Read the model definition and answer for the solid it produces. Units are mm, in the model's axes. Round coordinates to 2 decimals unless told otherwise and drop trailing zeros. Loops run counter-clockwise (first coordinate to the right, second up) from the corner with the lowest first, then second, coordinate; pieces in that order, holes last. Notation, with made-up numbers: M 84,-29 L 109,-29 A32 cw 109,9 Z; hole C 16.5,45 d3. An arc over 180 degrees is marked long. Write each question's results on one line, items separated by ' | '.
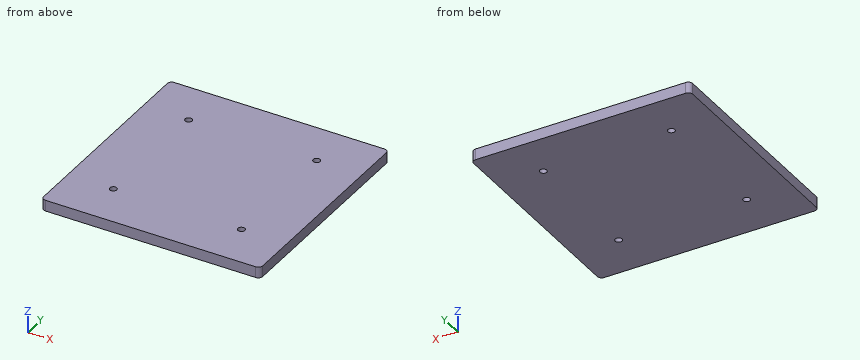
Autodesk Inventor part; units mm, degrees
ref_plane "YZ Plane" through (0, 0, 0) normal (1, 0, 0) x (0, 1, 0)
ref_plane "XZ Plane" through (0, 0, 0) normal (0, 1, 0) x (-1, 0, 0)
ref_plane "XY Plane" through (0, 0, 0) normal (0, 0, 1) x (1, 0, 0)
ref_plane "Plano de trabajo1" through (0, 0, 150) normal (0, 0, 1) x (1, 0, 0)
sketch "Boceto1" plane through (0, 0, 150) normal (0, 0, 1) x (1, 0, 0)
  line L0 (-96, 100) -> (96, 100)
  line L1 (100, 96) -> (100, -96)
  line L2 (96, -100) -> (-96, -100)
  line L3 (-100, -96) -> (-100, 96)
  line L4 (-100, 100) -> (100, -100) construction
  line L5 (100, 100) -> (-100, -100) construction
  arc A0 (100, 96) -> (96, 100) centre (96, 96) ccw
  arc A1 (-96, 100) -> (-100, 96) centre (-96, 96) ccw
  arc A2 (-100, -96) -> (-96, -100) centre (-96, -96) ccw
  arc A3 (96, -100) -> (100, -96) centre (96, -96) ccw
  circle A4 centre (58.5, 58.5) radius 3.175
  circle A5 centre (-58.5, 58.5) radius 3.175
  circle A6 centre (-58.5, -58.5) radius 3.175
  circle A7 centre (58.5, -58.5) radius 3.175
  point P0 (0, 0)
  dimension "d0" = 200
  dimension "d1" = 200
  dimension "d2" = 4
extrude "Extrusión1" add sketch "Boceto1" along normal blind 10
properties part number "TablaSoporte2" material "Madera (abedul)"
1. Find section A-A, the plane y = -58.5. Give the vertices of the cut face in (x, z) (3 decimals), then the cut area to 3 significant figures.
Completed:
outline: M -100,150 L -61.675,150 L -61.675,160 L -100,160 Z; M -55.325,150 L 55.325,150 L 55.325,160 L -55.325,160 Z; M 61.675,150 L 100,150 L 100,160 L 61.675,160 Z | area: 1,870 mm2
2. Find the intervals of material crossed by L1, parallel to Y at x = 58.5, z = 156 (3 decimals); L2, parallel to Y at x = 57, z = 152, in increasing order.
Completed:
L1: y = -100 to -61.675, -55.325 to 55.325, 61.675 to 100 | L2: y = -100 to -61.3, -55.7 to 55.7, 61.3 to 100
3. Given P1, Ø8.5, axis at x = 58.5, y = 58.5, coming from the -Z side; P2, Ø5.5, axis at x = -58.5, y = 58.5, coming from the -Z side, each flat-ended and moving along its own axis, determine where each tip first touches the part or whether it passes through.
Completed:
P1: stops at z = 150 | P2: passes through
